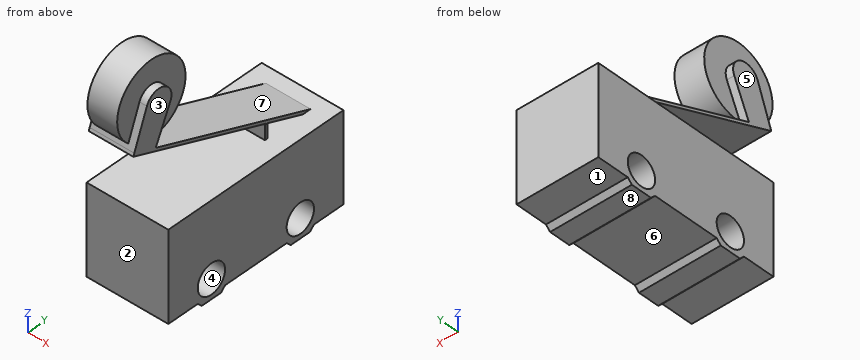
```python
from build123d import *

# Parameters (mm, degrees)
EXTRUDE_2_DEPTH      = 2.75
EXTRUDE_2_DEPTH_BACK = 2.75
SKETCH_1_R           = 1
EXTRUDE_3_DEPTH      = 1.5
EXTRUDE_3_DEPTH_BACK = 1.5
SKETCH_3_R           = 2.5
EXTRUDE_4_DEPTH      = 1


with BuildPart() as part:
    # 草图1 → 凸台-拉伸2 (new, two sides: drawn at the far end of the back side and taken through both)
    with BuildSketch(Plane(origin=(0, 0, 0), x_dir=(0, 0, -1), z_dir=(1, 0, 0)).offset(-EXTRUDE_2_DEPTH_BACK)):
        Polygon((0, 0), (6, 0), (6, -2.15), (6.3, -2.45), (6.3, -3.85), (6, -4.15), (6, -8.65), (6.3, -8.95), (6.3, -10.35), (6, -10.65), (6, -12.8), (0, -12.8), align=None)
        with Locations((5, -3.15)):
            Circle(SKETCH_1_R, mode=Mode.SUBTRACT)
        with Locations((5, -9.65)):
            Circle(SKETCH_1_R, mode=Mode.SUBTRACT)
    extrude(amount=EXTRUDE_2_DEPTH + EXTRUDE_2_DEPTH_BACK)

    # 草图2 → 凸台-拉伸3 (add, two sides: drawn at the far end of the back side and taken through both)
    with BuildSketch(Plane(origin=(0, 0, 0), x_dir=(0, 0, -1), z_dir=(1, 0, 0)).offset(-EXTRUDE_3_DEPTH_BACK)):
        with BuildLine():
            Line((0.187151005, -1.111689384), (-0.969179354, -4.18))
            Line((-0.969179354, -4.18), (-0.9, -4.18))
            Line((-0.9, -4.18), (0, -4.18))
            Line((0, -4.18), (0, -4.38))
            Line((0, -4.38), (-0.9, -4.38))
            ThreePointArc((-0.9, -4.38), (-0.982239003, -4.336892411), (-0.993575503, -4.244734928))
            Line((-0.993575503, -4.244734928), (-1.042296193, -4.374014774))
            Line((-1.042296193, -4.374014774), (-4.669966382, -14))
            Line((-4.669966382, -14), (-4.857117387, -13.929469856))
            Line((-4.857117387, -13.929469856), (-7.302366921, -13.007947681))
            ThreePointArc((-7.302366921, -13.007947681), (-7.831389963, -11.781984382), (-6.587549984, -11.296481041))
            Line((-6.587549984, -11.296481041), (-4.266871892, -12.363259556))
            Line((-4.266871892, -12.363259556), (0, -1.04115924))
            Line((0, -1.04115924), (0.187151005, -1.111689384))
        make_face()
    extrude(amount=EXTRUDE_3_DEPTH + EXTRUDE_3_DEPTH_BACK)

    # 草图3 → 凸台-拉伸4 (add, symmetric)
    with BuildSketch(Plane(origin=(0, 0, 0), x_dir=(0, 0, -1), z_dir=(1, 0, 0))):
        with Locations((-6.975125085, -12.139614863)):
            Circle(SKETCH_3_R)
    extrude(amount=EXTRUDE_4_DEPTH, both=True)


solid = part.part
```
For this review, take the finished solid that the model builds, in its own axes (mm). Face numbers are marked on the shaded views. A direction names the side the tool comes from. Round coordinates to 2 decimals unless told otherwise and drop trailing zeros. Write each loop counter-clockwise with the first axis right and the second up, starting at its lowest first coordinate (ties: lowest second). Pieces come first, ordered by that corner, then holes.
1) For line 1 along Y through (x, z) = (-1.25, -5); line 2 along Z through (x, y) = (-0.8, -9.25); line 3 along Z through (x, y) = (1.3, -3), list the stretches that pass through material, from the lowest coordinate up.
Answer below:
line 1: y = -12.8 to -10.65, -8.65 to -4.15, -2.15 to 0
line 2: z = -6.3 to -5.92, -4.08 to 0, 2.88 to 3.09
line 3: z = -6.3 to -5.99, -4.01 to 0, 0.52 to 0.74
2) Take a section at B-B on x = 1.3. Give the boundary of the cut face in (y, z), then the cut area to 3 significant figures.
Answer below:
outline: (-14, 4.67) - (-4.24, 0.99) arc R0.1 ccw to (-4.38, 0.9) - (-4.38, 0) - (-12.8, 0) - (-12.8, -6) - (-10.65, -6) - (-10.35, -6.3) - (-8.95, -6.3) - (-8.65, -6) - (-4.15, -6) - (-3.85, -6.3) - (-2.45, -6.3) - (-2.15, -6) - (0, -6) - (0, 0) - (-1.04, 0) - (-12.36, 4.27) - (-11.3, 6.59) arc R0.93 ccw (long way) to (-13.01, 7.3) - close; hole circle Ø2 at (-9.65, -5); hole (-4.18, 0) - (-1.61, 0) - (-4.18, 0.97) - close; hole circle Ø2 at (-3.15, -5)
area: 80.4 mm2
3) Take a section at C-C on x = -2.4. Give the boundary of the cut face in (y, z).
Answer below:
outline: (-12.8, -6) - (-10.65, -6) - (-10.35, -6.3) - (-8.95, -6.3) - (-8.65, -6) - (-4.15, -6) - (-3.85, -6.3) - (-2.45, -6.3) - (-2.15, -6) - (0, -6) - (0, 0) - (-12.8, 0) - close; hole circle Ø2 at (-9.65, -5); hole circle Ø2 at (-3.15, -5)
4) Take a section at D-D on y = -5. Give the boundary of the cut face in (x, z), then the cut area to 3 significant figures.
Answer below:
outline: (-2.75, -6) - (2.75, -6) - (2.75, 0) - (-2.75, 0) - close; (-1.5, 1.28) - (1.5, 1.28) - (1.5, 1.49) - (-1.5, 1.49) - close
area: 33.6 mm2
5) Machinability: for the marked faces 1, 2, 3, 4 and 5, which of the approach directions +Z, -Z, +X, -X, +Y, -Y give a long, thin tool a straight path to every point of the face, cutting with its end or side? Answer none if there is none.
Answer below:
face 1: -Z, +X, -X, +Y
face 2: -Z, +X, -X, -Y
face 3: +Z, +X, +Y, -Y
face 4: +X, -X
face 5: +Z, -X, +Y, -Y
6) Insertion check: pin 1 Ø3 at (x, z) = (-2, 5) entering from -Y; pin 2 Ø2.5 at (y, z) = (-11, 7.5) entering from +X; pin 3 Ø1.5 at (y, z) = (-12.5, 7) entering from -X. Each pin has a flat end and moves straight along its axis. Give the tip position at first contact, or say it passes through.
Answer below:
pin 1: stops at y = -14.49
pin 2: stops at x = 1.5
pin 3: stops at x = -1.5
7) Mouldability with a two-part tool opening along Y and no side actions: class the marked faces 6, 7 and 8 as +Y half, -Y half, draft (parallel to the pull), parting line (faces both ways), or undercut.
Answer below:
face 6: undercut
face 7: +Y half
face 8: draft
8) Take a section at A-A on z = -5. Give the boundary of the cut face in (x, y), then the cut area to 3 significant figures.
Answer below:
outline: (-2.75, -12.8) - (2.75, -12.8) - (2.75, -10.65) - (-2.75, -10.65) - close; (-2.75, -8.65) - (2.75, -8.65) - (2.75, -4.15) - (-2.75, -4.15) - close; (-2.75, -2.15) - (2.75, -2.15) - (2.75, 0) - (-2.75, 0) - close
area: 48.4 mm2
